from build123d import *

# Parameters (mm, degrees)
ESQUISSE1_R        = 7.55
ESQUISSE1_R_2      = 3
BOSS_EXTRU_1_DEPTH = 13


with BuildPart() as part:
    # Esquisse1 → Boss.-Extru.1 (new body)
    with BuildSketch(Plane.XY):
        with BuildLine():
            Line((93.987648188, -26), (93.940672922, -43.994779029))
            ThreePointArc((93.940672922, -43.994779029), (94.524607857, -45.412366464), (95.940666108, -46))
            Line((95.940666108, -46), (104, -46))
            ThreePointArc((104, -46), (105.36856155, -45.433123245), (105.935438305, -44.064561695))
            Line((105.935438305, -44.064561695), (105.935438305, 44.064561695))
            ThreePointArc((105.935438305, 44.064561695), (105.36856155, 45.433123245), (104, 46))
            Line((104, 46), (95.940666108, 46))
            ThreePointArc((95.940666108, 46), (94.524607857, 45.412366464), (93.940672922, 43.994779029))
            Line((93.940672922, 43.994779029), (93.987648188, 26))
            Line((93.987648188, 26), (87, 26))
            ThreePointArc((87, 26), (84.171572875, 24.828427125), (83, 22))
            Line((83, 22), (83, 20.508086384))
            ThreePointArc((83, 20.508086384), (81.828427125, 17.679659259), (79, 16.508086384))
            Line((79, 16.508086384), (15.30445081, 16.508086384))
            ThreePointArc((15.30445081, 16.508086384), (10.30445081, 17.847832346), (6.644196772, 21.508086384))
            Line((6.644196772, 21.508086384), (-25.203577824, 76.670050091))
            ThreePointArc((-25.203577824, 76.670050091), (-25.603179514, 79.705326271), (-23.739476208, 82.134151706))
            Line((-23.739476208, 82.134151706), (-22.447441117, 82.880108514))
            ThreePointArc((-22.447441117, 82.880108514), (-20.583737812, 85.308933949), (-20.983339502, 88.344210129))
            Line((-20.983339502, 88.344210129), (-24.477163596, 94.395690973))
            Line((-24.477163596, 94.395690973), (-8.869740188, 103.352398714))
            ThreePointArc((-8.869740188, 103.352398714), (-7.934040924, 104.566894919), (-8.13316448, 106.087054105))
            Line((-8.13316448, 106.087054105), (-12.162831426, 113.066641994))
            ThreePointArc((-12.162831426, 113.066641994), (-13.338041871, 113.968412685), (-14.806689318, 113.775061581))
            Line((-14.806689318, 113.775061581), (-91.128748987, 69.710499885))
            ThreePointArc((-91.128748987, 69.710499885), (-92.030519678, 68.53528944), (-91.837168574, 67.066641994))
            Line((-91.837168574, 67.066641994), (-87.807501628, 60.087054105))
            ThreePointArc((-87.807501628, 60.087054105), (-86.590566932, 59.154528454), (-85.070932735, 59.357619685))
            Line((-85.070932735, 59.357619685), (-69.510484592, 68.395690973))
            Line((-69.510484592, 68.395690973), (-66.016660498, 62.344210129))
            ThreePointArc((-66.016660498, 62.344210129), (-63.587835064, 60.480506824), (-60.552558883, 60.880108514))
            Line((-60.552558883, 60.880108514), (-59.260523792, 61.626065322))
            ThreePointArc((-59.260523792, 61.626065322), (-56.225247611, 62.025667012), (-53.796422176, 60.161963707))
            Line((-53.796422176, 60.161963707), (-21.948647581, 5))
            ThreePointArc((-21.948647581, 5), (-20.608901619, 0), (-21.948647581, -5))
            Line((-21.948647581, -5), (-53.796422176, -60.161963707))
            ThreePointArc((-53.796422176, -60.161963707), (-56.225247611, -62.025667012), (-59.260523792, -61.626065322))
            Line((-59.260523792, -61.626065322), (-60.552558883, -60.880108514))
            ThreePointArc((-60.552558883, -60.880108514), (-63.587835064, -60.480506824), (-66.016660498, -62.344210129))
            Line((-66.016660498, -62.344210129), (-69.510484592, -68.395690973))
            Line((-69.510484592, -68.395690973), (-85.070932735, -59.357619685))
            ThreePointArc((-85.070932735, -59.357619685), (-86.590566932, -59.154528455), (-87.807501628, -60.087054105))
            Line((-87.807501628, -60.087054105), (-91.837168574, -67.066641994))
            ThreePointArc((-91.837168574, -67.066641994), (-92.030519678, -68.53528944), (-91.128748987, -69.710499885))
            Line((-91.128748987, -69.710499885), (-14.806689318, -113.775061581))
            ThreePointArc((-14.806689318, -113.775061581), (-13.338041871, -113.968412685), (-12.162831426, -113.066641994))
            Line((-12.162831426, -113.066641994), (-8.13316448, -106.087054105))
            ThreePointArc((-8.13316448, -106.087054105), (-7.934040924, -104.566894919), (-8.869740188, -103.352398714))
            Line((-8.869740188, -103.352398714), (-24.477163596, -94.395690973))
            Line((-24.477163596, -94.395690973), (-20.983339502, -88.344210129))
            ThreePointArc((-20.983339502, -88.344210129), (-20.583737812, -85.308933949), (-22.447441117, -82.880108514))
            Line((-22.447441117, -82.880108514), (-23.739476208, -82.134151706))
            ThreePointArc((-23.739476208, -82.134151706), (-25.603179514, -79.705326271), (-25.203577824, -76.670050091))
            Line((-25.203577824, -76.670050091), (6.644196772, -21.508086384))
            ThreePointArc((6.644196772, -21.508086384), (10.30445081, -17.847832346), (15.30445081, -16.508086384))
            Line((15.30445081, -16.508086384), (79, -16.508086384))
            ThreePointArc((79, -16.508086384), (81.828427125, -17.679659259), (83, -20.508086384))
            Line((83, -20.508086384), (83, -22))
            ThreePointArc((83, -22), (84.171572875, -24.828427125), (87, -26))
            Line((87, -26), (93.987648188, -26))
        make_face()
        with Locations(Location((0, 0, 0), (0, 0, 180))):
            Circle(ESQUISSE1_R, mode=Mode.SUBTRACT)
        with Locations(Location((20, 0, 0), (0, 0, 180))):
            Circle(ESQUISSE1_R_2, mode=Mode.SUBTRACT)
        with Locations(Location((40, 0, 0), (0, 0, 180))):
            Circle(ESQUISSE1_R_2, mode=Mode.SUBTRACT)
        with Locations(Location((60, 0, 0), (0, 0, 180))):
            Circle(ESQUISSE1_R_2, mode=Mode.SUBTRACT)
        with Locations(Location((70, 0, 0), (0, 0, 180))):
            Circle(ESQUISSE1_R_2, mode=Mode.SUBTRACT)
        with Locations(Location((50, 0, 0), (0, 0, 180))):
            Circle(ESQUISSE1_R_2, mode=Mode.SUBTRACT)
        with Locations(Location((30, 0, 0), (0, 0, 180))):
            Circle(ESQUISSE1_R_2, mode=Mode.SUBTRACT)
        with Locations(Location((-35, -60.621778265, 0), (0, 0, 180))):
            Circle(ESQUISSE1_R_2, mode=Mode.SUBTRACT)
        with Locations(Location((-30, -51.961524227, 0), (0, 0, 180))):
            Circle(ESQUISSE1_R_2, mode=Mode.SUBTRACT)
        with Locations(Location((-25, -43.301270189, 0), (0, 0, 180))):
            Circle(ESQUISSE1_R_2, mode=Mode.SUBTRACT)
        with Locations(Location((-15, -25.980762114, 0), (0, 0, 180))):
            Circle(ESQUISSE1_R_2, mode=Mode.SUBTRACT)
        with Locations(Location((-10, -17.320508076, 0), (0, 0, 180))):
            Circle(ESQUISSE1_R_2, mode=Mode.SUBTRACT)
        with Locations(Location((-20, -34.641016151, 0), (0, 0, 180))):
            Circle(ESQUISSE1_R_2, mode=Mode.SUBTRACT)
        with Locations(Location((-35, 60.621778265, 0), (0, 0, 180))):
            Circle(ESQUISSE1_R_2, mode=Mode.SUBTRACT)
        with Locations(Location((-30, 51.961524227, 0), (0, 0, 180))):
            Circle(ESQUISSE1_R_2, mode=Mode.SUBTRACT)
        with Locations(Location((-25, 43.301270189, 0), (0, 0, 180))):
            Circle(ESQUISSE1_R_2, mode=Mode.SUBTRACT)
        with Locations(Location((-15, 25.980762114, 0), (0, 0, 180))):
            Circle(ESQUISSE1_R_2, mode=Mode.SUBTRACT)
        with Locations(Location((-10, 17.320508076, 0), (0, 0, 180))):
            Circle(ESQUISSE1_R_2, mode=Mode.SUBTRACT)
        with Locations(Location((-20, 34.641016151, 0), (0, 0, 180))):
            Circle(ESQUISSE1_R_2, mode=Mode.SUBTRACT)
    extrude(amount=BOSS_EXTRU_1_DEPTH)


solid = part.part
Work out the finished part from the listing and answer in its coordinate system (mm). A direction names the side the tool comes from. Coordinates: 2 decimals unless noted, no trailing zeros. Order: outer loops, then holes, each group sorted by start corner. A loop starts at its lowest first (then second) coordinate and runs counter-clockwise, first axis right, second up. Notation, with made-up numbers: (31.5, 30) - (54.5, 30) arc R10 ccw to (54.5, 40) - close; hole circle Ø1 at (-7, 49). An arc over 180 degrees is marked (long way). Put each result on its own line as item: value. Start each with the question number.
1) Find section A-A (x = 70). Give the vertices of the cut face in (y, z).
2) For faces 1 (the cylindrical face through (10.241, -17.885, 6.409)), 2 (the flat face through (-22.755, -91.412, 6.409)), 3 (the flat face through (-89.794, -63.528, 6.409)), determine the directions among +Z, -Z, +X, -X, +Y, -Y from which every point of the face is accessible in a straight line to the end or side of a thin tool.
3) Find section B-B (z = 10.75). State how many separate pieces and enclosed holes the cut face has, plus the area to 3 significant figures.
4) Flat-ended cylindrical pins translate along their axes: pin 1 (3.5 mm diameter, centred on x = 50, y = 0, fed in from +Z); pin 2 (1 mm diameter, centred on x = -68, z = 9, fed in from +Y); pin 3 (1.5 mm diameter, centred on y = -29.5, z = 6.5, fed in from -X); pin 4 (6.5 mm diameter, centred on x = 99, z = 9, fed in from +Y). Find the tip coordinate at first contact, or state that the pin passes through.
5) For a pull along X with two mould halves and no side action, classify faces 4 (the flat face through (6, -8, 13)), 5 (the cylindrical face through (-12.79, -28.01, 6.41)), 6 (the cylindrical face through (-25.59, -79.75, 6.41)) as released by +X, released by -X, zero draft, split by the parting line, or undercut.
6) Find the intervals of material crossed by line 1 (X direction, y = 36, z = 12.25); line 2 (X direction, y = -33.5, z = 10); line 3 (Y direction, x = -15, z = 10), in increasing order. Write a range as from..to.
7) Find section C-C (x = 0). Give the vertices of the cut face in (y, z).
Results list:
1. outline: (-16.51, 0) - (-3, 0) - (-3, 13) - (-16.51, 13) - close; (3, 0) - (16.51, 0) - (16.51, 13) - (3, 13) - close
2. face 1: +Z, -Z, -Y
2. face 2: +Z, -Z, +X
2. face 3: +Z, -Z, -X
3. separate pieces: 1
3. enclosed holes: 19
3. area: 12,100 mm^2
4. pin 1: passes through
4. pin 2: stops at y = 83.35
4. pin 3: stops at x = -36.53
4. pin 4: stops at y = 46
5. face 4: zero draft
5. face 5: undercut
5. face 6: released by +X
6. line 1: x = -39.85..-22.67, -17.33..-1.72, 93.96..105.94
6. line 2: x = -38.4..-22.77, -17.23..-0.28, 93.97..105.94
6. line 3: y = -113.66..-99.83, -59..-28.98, -22.98..22.98, 28.98..59, 99.83..113.66
7. outline: (-33.02, 0) - (-7.55, 0) - (-7.55, 13) - (-33.02, 13) - close; (7.55, 0) - (33.02, 0) - (33.02, 13) - (7.55, 13) - close
